```python
from build123d import *

# Parameters (mm, degrees)
SALIENTE_EXTRUIR15_DEPTH = 3
SALIENTE_EXTRUIR16_REACH = 85.791
CHAFL_N1_SIZE            = 8
CHAFL_N1_SIZE_2          = 2.205109306
CHAFL_N2_SIZE            = 2.205109306
CHAFL_N2_SIZE_2          = 8
SALIENTE_EXTRUIR17_DEPTH = 3
SALIENTE_EXTRUIR18_DEPTH = 102.97
CROQUIS28_R              = 1.825
CORTAR_EXTRUIR6_DEPTH    = 283.951050372
SALIENTE_EXTRUIR19_DEPTH = 100
CROQUIS30_R              = 1.65
CORTAR_EXTRUIR7_DEPTH    = 283.951050372
CORTAR_EXTRUIR9_REACH    = 302.941
CORTAR_EXTRUIR10_START   = -40.653307
CROQUIS34_R              = 2.5
CORTAR_EXTRUIR10_DEPTH   = 35
CROQUIS35_W              = 41.244426213
CROQUIS35_H              = 6
CORTAR_EXTRUIR11_DEPTH   = 17
CROQUIS36_W              = 41.244426207
CROQUIS36_H              = 6
CORTAR_EXTRUIR12_DEPTH   = 17
CROQUIS37_W              = 139.956448948
CROQUIS37_H              = 12
CORTAR_EXTRUIR13_DEPTH   = 3
CROQUIS39_W              = 88.97
CROQUIS39_H              = 15
CROQUIS39_H_2            = 10
CORTAR_EXTRUIR14_DEPTH   = 353.231866742
CHAFL_N4_SIZE            = 3.639702343
CHAFL_N4_SIZE_2          = 10


with BuildPart() as part:
    # Croquis22 → Saliente-Extruir15 (new body)
    with BuildSketch(Plane.XY):
        Polygon((-54, 0), (54, 0), (35.527349199, 64), (-35.527349199, 64), align=None)
    extrude(amount=SALIENTE_EXTRUIR15_DEPTH)

    # Saliente-Extruir16: up to this face of the body (flat: up to its plane)
    saliente_extruir16_end = Plane(part.part.faces().sort_by_distance((0, 0, 1.5))[0])
    # Croquis23 → Saliente-Extruir16 (add, up to the picked face)
    with BuildSketch(Plane(origin=(0, 64, 0), x_dir=(1, 0, 0), z_dir=(0, 1, 0)), mode=Mode.PRIVATE) as saliente_extruir16_sk1:
        Polygon((108.068224474, 30.82636567), (108.068224474, 254.28636567), (105.068224474, 254.28636567), (105.068224474, 32.737576452), (34.862265211, 0), (44.7636746, -3), align=None)
    saliente_extruir16_tool1 = split(extrude(saliente_extruir16_sk1.sketch, amount=-SALIENTE_EXTRUIR16_REACH, mode=Mode.PRIVATE), bisect_by=saliente_extruir16_end, keep=Keep.BOTH, mode=Mode.PRIVATE)
    # Croquis23 → Saliente-Extruir16 (add, up to the picked face)
    with BuildSketch(Plane(origin=(0, 64, 0), x_dir=(1, 0, 0), z_dir=(0, 1, 0)), mode=Mode.PRIVATE) as saliente_extruir16_sk2:
        Polygon((-44.7636746, -3), (-108.068224474, 30.82636567), (-108.068224474, 254.28636567), (-105.068224474, 254.28636567), (-105.068224474, 32.737576452), (-34.862265211, 0), align=None)
    saliente_extruir16_tool2 = split(extrude(saliente_extruir16_sk2.sketch, amount=-SALIENTE_EXTRUIR16_REACH, mode=Mode.PRIVATE), bisect_by=saliente_extruir16_end, keep=Keep.BOTH, mode=Mode.PRIVATE)
    add(saliente_extruir16_tool1.solids().sort_by(Axis((105.393241, 64, -142.556366), (0, -1, 0)))[0])
    add(saliente_extruir16_tool2.solids().sort_by(Axis((-75.155279, 64, -16.272473), (0, -1, 0)))[0])

    # Chaflán1
    # the kernel refuses this chamfer: 8, 2.205109306 mm, written as the material it adds along each edge
    with BuildSketch(Plane(origin=(-50.503325007, 12.114514694, 4.739040428), x_dir=(-0.919298302367056, 0.2887303877017334, 0.267442319917128), z_dir=(0.2763409092722936, 0.9574055388276669, -0.0837277497886264))) as chafl_n1_piece_1_section:
        Polygon((CHAFL_N1_SIZE * 0.999943641705, CHAFL_N1_SIZE * 0.0106166574103), (CHAFL_N1_SIZE_2 * 0.268384707917, CHAFL_N1_SIZE_2 * 0.963311812656), (0, 0), align=None)
    chafl_n1_piece_1 = extrude(amount=74.96402277, mode=Mode.PRIVATE)
    chafl_n1_piece_1 = split(chafl_n1_piece_1, bisect_by=Plane(origin=(-40.189826284, 64, 2.253573464), z_dir=(0, -1, 0)), keep=Keep.TOP, mode=Mode.PRIVATE)
    chafl_n1_piece_1 = split(chafl_n1_piece_1, bisect_by=Plane(origin=(-40.189826284, 55.464802275, 3), z_dir=(0, 0, -1)), keep=Keep.TOP, mode=Mode.PRIVATE)
    add(chafl_n1_piece_1)

    # Chaflán2
    # the kernel refuses this chamfer: 8, 2.205109306 mm, written as the material it adds along each edge
    with BuildSketch(Plane(origin=(50.503325007, 12.114514694, 4.739040428), x_dir=(-0.1610184044916604, 0.03976595413217484, 0.9861499593403216), z_dir=(-0.27634090927229366, 0.957405538827667, -0.08372774978862642))) as chafl_n2_piece_1_section:
        Polygon((CHAFL_N2_SIZE * 0.989624861472, CHAFL_N2_SIZE * 0.143675444677), (CHAFL_N2_SIZE_2 * 0.137719182616, CHAFL_N2_SIZE_2 * 0.990471315455), (0, 0), align=None)
    chafl_n2_piece_1 = extrude(amount=74.96402277, mode=Mode.PRIVATE)
    chafl_n2_piece_1 = split(chafl_n2_piece_1, bisect_by=Plane(origin=(40.189826284, 55.464802275, 3), z_dir=(0, 0, -1)), keep=Keep.TOP, mode=Mode.PRIVATE)
    chafl_n2_piece_1 = split(chafl_n2_piece_1, bisect_by=Plane(origin=(40.189826284, 64, 2.253573464), z_dir=(0, -1, 0)), keep=Keep.TOP, mode=Mode.PRIVATE)
    add(chafl_n2_piece_1)

    # Croquis24 → Saliente-Extruir17 (add)
    with BuildSketch(Plane(origin=(0, 64, 0), x_dir=(1, 0, 0), z_dir=(0, 1, 0))):
        with BuildLine():
            Line((-108.068224474, 93.00636567), (-108.068224474, 30.82636567))
            Line((-108.068224474, 30.82636567), (-44.7636746, -3))
            Line((-44.7636746, -3), (44.7636746, -3))
            Line((44.7636746, -3), (108.068224474, 30.82636567))
            Line((108.068224474, 30.82636567), (108.068224474, 93.00636567))
            ThreePointArc((108.068224474, 93.00636567), (0, 69.74), (-108.068224474, 93.00636567))
        make_face()
    extrude(amount=-SALIENTE_EXTRUIR17_DEPTH)

    # Croquis25 → Saliente-Extruir18 (add)
    with BuildSketch(Plane(origin=(0, 0, -254.28636567), x_dir=(-1, 0, 0), z_dir=(0, 0, -1))):
        Polygon((-108.068224474, 64), (-79.978224474, 112.653307185), (79.978224474, 112.653307185), (108.068224474, 64), (105.068224474, 63.196152423), (78.246173666, 109.653307185), (-78.246173666, 109.653307185), (-105.068224474, 63.196152423), align=None)
    extrude(amount=-SALIENTE_EXTRUIR18_DEPTH)

    # Croquis28 → Cortar-Extruir6 (cut, through all)
    with BuildSketch(Plane.XZ.offset(-61)):
        with Locations(Location((-0.001775526, -60.825, 0), (0, 0, 270))):
            Circle(CROQUIS28_R)
    extrude(amount=-CORTAR_EXTRUIR6_DEPTH, mode=Mode.SUBTRACT)

    # Croquis29 → Saliente-Extruir19 (add)
    with BuildSketch(Plane(origin=(0, 0, -254.28636567), x_dir=(-1, 0, 0), z_dir=(0, 0, -1))):
        Polygon((-105.068224474, 61), (-90.068224474, 61), (-90.068224474, 89.176914536), (-105.068224474, 63.196152423), align=None)
        Polygon((105.068224474, 61), (105.068224474, 63.196152423), (90.068224474, 89.176914536), (90.068224474, 61), align=None)
    extrude(amount=-SALIENTE_EXTRUIR19_DEPTH)

    # Croquis30 → Cortar-Extruir7 (cut, through all)
    with BuildSketch(Plane.XZ.offset(-61)):
        with Locations(Location((94.857727132, -169.052479414, 0), (0, 0, 270))):
            Circle(CROQUIS30_R)
        with Locations(Location((94.857727132, -229.296905627, 0), (0, 0, 270))):
            Circle(CROQUIS30_R)
        with Locations(Location((-94.857727132, -229.296905627, 0), (0, 0, 180))):
            Circle(CROQUIS30_R)
        with Locations(Location((-94.857727132, -169.052479414, 0), (0, 0, 180))):
            Circle(CROQUIS30_R)
    extrude(amount=-CORTAR_EXTRUIR7_DEPTH, mode=Mode.SUBTRACT)

    # Cortar-Extruir9: up to this face of the body (flat: up to its plane)
    cortar_extruir9_end = Plane(part.part.faces().sort_by_distance((95.429754053, 70.445236449, -154.28636567))[0])
    # Croquis33 → Cortar-Extruir9 (cut, up to the picked face)
    with BuildSketch(Plane(origin=(0, 0, -254.28636567), x_dir=(-1, 0, 0), z_dir=(0, 0, -1)), mode=Mode.PRIVATE) as cortar_extruir9_sk1:
        Polygon((-90.068224474, 61), (-90.068224474, 72), (-99.985320705, 72), (-106.336173666, 61), align=None)
    cortar_extruir9_tool1 = split(extrude(cortar_extruir9_sk1.sketch, amount=-CORTAR_EXTRUIR9_REACH, mode=Mode.PRIVATE), bisect_by=cortar_extruir9_end, keep=Keep.BOTH, mode=Mode.PRIVATE)
    # Croquis33 → Cortar-Extruir9 (cut, up to the picked face)
    with BuildSketch(Plane(origin=(0, 0, -254.28636567), x_dir=(-1, 0, 0), z_dir=(0, 0, -1)), mode=Mode.PRIVATE) as cortar_extruir9_sk2:
        Polygon((99.985320705, 72), (106.336173666, 61), (90.068224474, 61), (90.068224474, 72), align=None)
    cortar_extruir9_tool2 = split(extrude(cortar_extruir9_sk2.sketch, amount=-CORTAR_EXTRUIR9_REACH, mode=Mode.PRIVATE), bisect_by=cortar_extruir9_end, keep=Keep.BOTH, mode=Mode.PRIVATE)
    add(cortar_extruir9_tool1.solids().sort_by(Axis((96.742846, 66.055348, -254.286366), (0, 0, 1)))[0], mode=Mode.SUBTRACT)
    add(cortar_extruir9_tool2.solids().sort_by(Axis((-96.742846, 66.055348, -254.286366), (0, 0, 1)))[0], mode=Mode.SUBTRACT)

    # Croquis34 → Cortar-Extruir10 (cut)
    with BuildSketch(Plane.XZ.offset(-72).offset(CORTAR_EXTRUIR10_START)):
        with Locations(Location((94.857727132, -169.052479414, 0), (0, 0, 90))):
            Circle(CROQUIS34_R)
        with Locations(Location((94.857727132, -229.296905627, 0), (0, 0, 90))):
            Circle(CROQUIS34_R)
        with Locations(Location((-94.860104661, -169.05116859, 0), (0, 0, 90))):
            Circle(CROQUIS34_R)
        with Locations(Location((-94.860937159, -229.295594797, 0), (0, 0, 90))):
            Circle(CROQUIS34_R)
    extrude(amount=CORTAR_EXTRUIR10_DEPTH, mode=Mode.SUBTRACT)

    # Croquis35 → Cortar-Extruir11 (cut)
    with BuildSketch(Plane(origin=(108.763981276, 62.794913868, 0), x_dir=(0, 0, -1), z_dir=(0.8660254037844364, 0.5000000000000041, 0))):
        with Locations((199.174692521, 34.754013605)):
            Rectangle(CROQUIS35_W, CROQUIS35_H)
        with Locations((199.174692521, 45.299013605)):
            Rectangle(CROQUIS35_W, CROQUIS35_H)
        with Locations((199.174692521, 24.209013605)):
            Rectangle(CROQUIS35_W, CROQUIS35_H)
        with Locations((199.174692521, 13.664013605)):
            Rectangle(CROQUIS35_W, CROQUIS35_H)
    extrude(amount=-CORTAR_EXTRUIR11_DEPTH, mode=Mode.SUBTRACT)

    # Croquis36 → Cortar-Extruir12 (cut)
    with BuildSketch(Plane(origin=(-108.763981276, 62.794913868, 0), x_dir=(0, 0, 1), z_dir=(-0.8660254037844363, 0.500000000000004, 0))):
        with Locations((-199.173381694, 33.498068951)):
            Rectangle(CROQUIS36_W, CROQUIS36_H)
        with Locations((-199.173381694, 44.880365387)):
            Rectangle(CROQUIS36_W, CROQUIS36_H)
        Polygon((-219.795070879, 19.114529475), (-219.795432544, 25.114529465), (-178.551006411, 25.117015574), (-178.550644747, 19.117015585), align=None)
        Polygon((-219.794384783, 7.73223306), (-178.549958651, 7.734719169), (-178.550320316, 13.734719158), (-219.794746448, 13.732233049), align=None)
    extrude(amount=-CORTAR_EXTRUIR12_DEPTH, mode=Mode.SUBTRACT)

    # Croquis37 → Cortar-Extruir13 (cut)
    with BuildSketch(Plane(origin=(0, 112.653307185, 0), x_dir=(1, 0, 0), z_dir=(0, 1, 0))):
        with Locations((0, 241.41511567)):
            Rectangle(CROQUIS37_W, CROQUIS37_H)
        with Locations((0, 215.67261567)):
            Rectangle(CROQUIS37_W, CROQUIS37_H)
        with Locations((0, 189.93011567)):
            Rectangle(CROQUIS37_W, CROQUIS37_H)
        with Locations((0, 164.18761567)):
            Rectangle(CROQUIS37_W, CROQUIS37_H)
    extrude(amount=-CORTAR_EXTRUIR13_DEPTH, mode=Mode.SUBTRACT)

    # Croquis39 → Cortar-Extruir14 (cut, through all)
    with BuildSketch(Plane.ZY.offset(108.068224474)):
        with Locations((-202.80136567, 33.877807024)):
            Rectangle(CROQUIS39_W, CROQUIS39_H)
        with Locations((-202.80136567, 5)):
            Rectangle(CROQUIS39_W, CROQUIS39_H_2)
    extrude(amount=-CORTAR_EXTRUIR14_DEPTH, mode=Mode.SUBTRACT)

    # Chaflán4
    # the kernel refuses this chamfer: 10, 3.639702343 mm, written as the material it takes off along each edge
    with BuildSketch(Plane(origin=(61.194082129, -24.924482209, 3), x_dir=(-0.9560553519940534, -0.27595119786771466, 0.0990409022520496), z_dir=(-0.27731465330238175, 0.9607791541575931, 0))) as chafl_n4_piece_1_section:
        Polygon((CHAFL_N4_SIZE * 0.995083363089, -CHAFL_N4_SIZE * 0.0990409022429), (-CHAFL_N4_SIZE_2 * 0.099040902252, -CHAFL_N4_SIZE_2 * 0.995083363182), (0, 0), align=None)
    chafl_n4_piece_1 = extrude(amount=85.19019596, mode=Mode.PRIVATE)
    chafl_n4_piece_1 = split(chafl_n4_piece_1, bisect_by=Plane(origin=(49.101684897, 9.648205997, 0.682013017), z_dir=(0.47128163735993633, 0, 0.881982776638715)), keep=Keep.TOP, mode=Mode.PRIVATE)
    add(chafl_n4_piece_1, mode=Mode.SUBTRACT)
    with BuildSketch(Plane(origin=(-37.569592471, 56.924482209, 3), x_dir=(0.9560553519940533, -0.27595119786771466, 0.09904090225204958), z_dir=(-0.27731465330238175, -0.9607791541575931, 0))) as chafl_n4_piece_2_section:
        Polygon((CHAFL_N4_SIZE * 0.995083363089, -CHAFL_N4_SIZE * 0.0990409022429), (-CHAFL_N4_SIZE_2 * 0.0990409022521, -CHAFL_N4_SIZE_2 * 0.995083363182), (0, 0), align=None)
    chafl_n4_piece_2 = extrude(amount=85.19019596, mode=Mode.PRIVATE)
    chafl_n4_piece_2 = split(chafl_n4_piece_2, bisect_by=Plane(origin=(-49.101684897, 9.648205997, 0.682013017), z_dir=(-0.47128163735993633, 0, 0.881982776638715)), keep=Keep.TOP, mode=Mode.PRIVATE)
    add(chafl_n4_piece_2, mode=Mode.SUBTRACT)


solid = part.part
```
Check sheet for the modelled part. Datum: model origin and axes. Units: mm. A direction names the side the tool comes from. Round coordinates to 2 decimals unless told otherwise and drop trailing zeros. Loops run counter-clockwise (first coordinate to the right, second up) from the corner with the lowest first, then second, coordinate; pieces in that order, holes last. Notation, with made-up numbers: (39, 66.25) - (60, 66.25) arc R25 cw to (60, 101.25) - close; hole circle Ø4 at (28, -29.5). An arc over 180 degrees is marked (long way). Answer as a JSON object with one key per item and string values. Group by question number.
Q1. Set-up check for faces 1 (the face through (-1, 109.653, -204)), 2 (the face through (-91, 91, -219.796)), 3 (the face through (93, 77, -154.286)): record each of +Z, -Z, +X, -X, +Y, -Y from which the full face is reachable in a straight line by a thin tool's end or side.
Q2. Sectioned sample at B-B, the plane z = -114.5. Enter the section's corners in (x, y).
Q3. Gauge pin test, flat ends, axial feed: P1, Ø6.5, axis at x = 94.86, z = -229.3, coming from the -Y side; P2, Ø1.4, axis at x = 105.5, z = -201, coming from the +Y side; P3, Ø1.5, axis at x = -6.5, y = 110.5, coming from the +Z side. Record the tip position at first contact, or that the pin passes through.
Q4. Scan lines: line 1 along X through (y, z) = (43, -59); line 2 along Y through (x, z) = (93, -232); line 3 along Y through (x, z) = (20, -38.5). Record each from-to range of solid material in increasing order. Write a range as [from, to].
Q5. Sectioned sample at A-A, the plane z = -163. Count the separate pieces of the cut face and the enclosed holes in it, plus the area to 3 significant figures.
Q6. Mould release check, pull along Z, two halves, no side actions. Record for faces 4 (the face through (1, 32, 3)), 5 (the face through (98, 73, -219.797)), 6 (the face through (-95, 72, -205)): released by +Z, released by -Z, zero draft, split by the parting line, or undercut.
Q7. Sectioned sample at D-D, the plane z = -40. Enter the section's corners in (x, y), plus the area to 3 significant figures.
Q8. Sectioned sample at C-C, the plane x = -14.5. Enter the section's corners in (y, z).
Solution:
{
 "1": {"face 1": "+Z, -Z, -Y", "face 2": "none", "face 3": "+Z, -Y"},
 "2": {"outline": "(-108.07, 0) - (-105.07, 0) - (-105.07, 64) - (-108.07, 64) - close; (105.07, 0) - (108.07, 0) - (108.07, 64) - (105.07, 64) - close"},
 "3": {"P1": "stops at y = 72", "P2": "stops at y = 69.66", "P3": "stops at z = -151.32"},
 "4": {"line 1": "x = [-108.07, -105.07], [105.07, 108.07]", "line 2": "y = [72, 90.1]", "line 3": "y = [61, 64]"},
 "5": {"separate pieces": "4", "enclosed holes": "0", "area": "783 mm²"},
 "6": {"face 4": "released by +Z", "face 5": "undercut", "face 6": "zero draft"},
 "7": {"outline": "(-108.07, 0) - (-105.07, 0) - (-105.07, 61) - (105.07, 61) - (105.07, 0) - (108.07, 0) - (108.07, 64) - (-108.07, 64) - close", "area": "1,010 mm²"},
 "8": {"outline": "(0, 0) - (61, 0) - (61, -70.14) - (64, -70.14) - (64, 3) - (0, 3) - close; (109.65, -254.29) - (112.65, -254.29) - (112.65, -247.42) - (109.65, -247.42) - close; (109.65, -235.42) - (112.65, -235.42) - (112.65, -221.67) - (109.65, -221.67) - close; (109.65, -209.67) - (112.65, -209.67) - (112.65, -195.93) - (109.65, -195.93) - close; (109.65, -183.93) - (112.65, -183.93) - (112.65, -170.19) - (109.65, -170.19) - close; (109.65, -158.19) - (112.65, -158.19) - (112.65, -151.32) - (109.65, -151.32) - close"}
}
